Could you check a few things on this model? Use its own coordinates, in mm. Coordinates: 2 decimals unless noted, no trailing zeros. Order: outer loops, then holes, each group sorted by start corner. A loop starts at its lowest first (then second) coordinate and runs counter-clockwise, first axis right, second up. Notation, with made-up numbers: (58.5, -17) - (96.5, -17) arc R22 cw to (96.5, 10) - close; hole circle Ø1 at (56.25, 81). An arc over 180 degrees is marked (long way). Answer as a JSON object with one key per item and string values. Group by question number.
(1) Imagine slicing it at C-C, the plane x = 60. Write out the boundary of the cut face in (y, z), and give its area (3 significant figures).
(2) Please list where these lines run through material, in increasing order: probe 1 along X at (y, z) = (9.5, 2.1); probe 2 along Y at (x, z) = (30, 1.6); probe 3 along X at (y, z) = (-3.5, 2.4).
(3) Imagine slicing it at A-A, the plane x = 30. Write out the boundary of the cut face in (y, z).
(4) Imagine slicing it at B-B, the plane z = 1.7. Write out the boundary of the cut face in (x, y).
(5) Will these pins go through, and if not, where does the flat tip stop? P1, Ø1.5, axis at y = -21, z = 1, coming from the -X side; P2, Ø1.5, axis at x = 23, z = 2, coming from the -Y side.
(6) Imagine slicing it at D-D, the plane y = -33. Write out the boundary of the cut face in (x, z), and give its area (3 significant figures).
from build123d import *

# Parameters (mm, degrees)
SKETCH1_R           = 3
BOSS_EXTRUDE1_DEPTH = 3


with BuildPart() as part:
    # Sketch1 → Boss-Extrude1 (new body)
    with BuildSketch(Plane.XY):
        with BuildLine():
            Line((77.087645862, 14.761424984), (61.884850067, -0.441370812))
            Line((61.884850067, -0.441370812), (91.229781486, -29.786302231))
            Line((91.229781486, -29.786302231), (82.534788155, -38.481295563))
            ThreePointArc((82.534788155, -38.481295563), (73.691938632, -33.074158425), (67.599954135, -24.688405948))
            ThreePointArc((67.599954135, -24.688405948), (60.573216822, -16.61605207), (50.302224608, -13.608619059))
            Line((50.302224608, -13.608619059), (10.897118181, -13.608619059))
            ThreePointArc((10.897118181, -13.608619059), (7.888998842, -13.847714786), (4.956418896, -14.558997838))
            ThreePointArc((4.956418896, -14.558997838), (-21.031882132, 1.283456288), (-1.283000467, 24.442834864))
            Line((-1.283000467, 24.442834864), (88.716999533, 24.442834864))
            ThreePointArc((88.716999533, 24.442834864), (89.976795131, 24.200731926), (91.057113295, 23.508914432))
            Line((91.057113295, 23.508914432), (109.912759821, 5.607389522))
            ThreePointArc((109.912759821, 5.607389522), (113.808768074, 0.948896759), (116.541784176, -4.474299542))
            Line((116.541784176, -4.474299542), (106.432577282, -14.583506436))
            Line((106.432577282, -14.583506436), (77.087645862, 14.761424984))
        make_face()
        with Locations((30, 7.5)):
            Circle(SKETCH1_R, mode=Mode.SUBTRACT)
        with Locations((-1.283000467, 4.442834864)):
            Circle(SKETCH1_R, mode=Mode.SUBTRACT)
        with Locations((60, 7.5)):
            Circle(SKETCH1_R, mode=Mode.SUBTRACT)
    extrude(amount=BOSS_EXTRUDE1_DEPTH)


solid = part.part
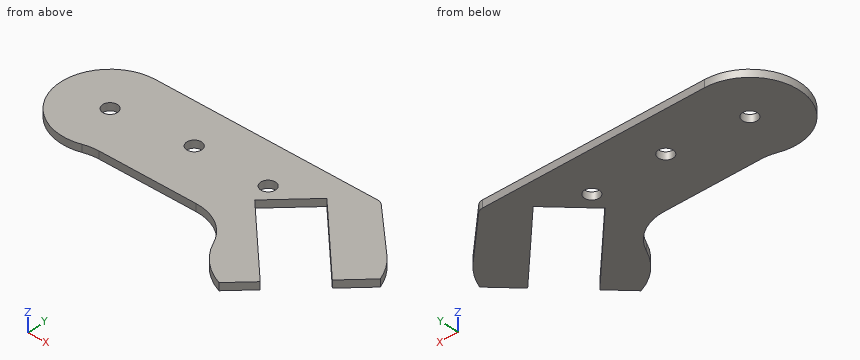
Result set:
{
 "1": {"outline": "(-16.26, 0) - (4.5, 0) - (4.5, 3) - (-16.26, 3) - close; (10.5, 0) - (24.44, 0) - (24.44, 3) - (10.5, 3) - close", "area": "104 mm^2"},
 "2": {"probe 1": "x = -20.63 to 27.76, 32.24 to 57.76, 62.24 to 71.83, 82.35 to 105.81", "probe 2": "y = -13.61 to 4.5, 10.5 to 24.44", "probe 3": "x = -19.64 to 64.94, 95.35 to 116.16"},
 "3": {"outline": "(-13.61, 0) - (4.5, 0) - (4.5, 3) - (-13.61, 3) - close; (10.5, 0) - (24.44, 0) - (24.44, 3) - (10.5, 3) - close"},
 "4": {"outline": "(-1.28, 24.44) arc R20 ccw (long way) to (4.96, -14.56) arc R19.04 cw to (10.9, -13.61) - (50.3, -13.61) arc R19.04 cw to (67.6, -24.69) arc R26.5 ccw to (82.53, -38.48) - (91.23, -29.79) - (61.88, -0.44) - (77.09, 14.76) - (106.43, -14.58) - (116.54, -4.47) arc R26.5 ccw to (109.91, 5.61) - (91.06, 23.51) arc R3.4 ccw to (88.72, 24.44) - close; hole circle Ø6 at (-1.28, 4.44); hole circle Ø6 at (30, 7.5); hole circle Ø6 at (60, 7.5)"},
 "5": {"P1": "stops at x = 64.75", "P2": "stops at y = -13.61"},
 "6": {"outline": "(73.61, 0) - (88.02, 0) - (88.02, 3) - (73.61, 3) - close", "area": "43.2 mm^2"}
}
